For this review, take the finished solid that the model builds, in its own axes (mm). Face numbers are marked on the shaded views. A direction names the side the tool comes from. Give positions to 0.01 mm unless a question says otherwise; leave off trailing zeros. Write each loop counter-clockwise with the first axis right and the second up, starting at its lowest first coordinate (ties: lowest second). Pieces come first, ordered by that corner, then holes. Notation, with made-up numbers: (24.5, -28) -> (43.5, -28) arc R19 ccw to (43.5, -19) -> close; hole circle Ø5 at (39.25, 53.25). An arc over 180 degrees is marked (long way). Answer as CSV lines item,"result".
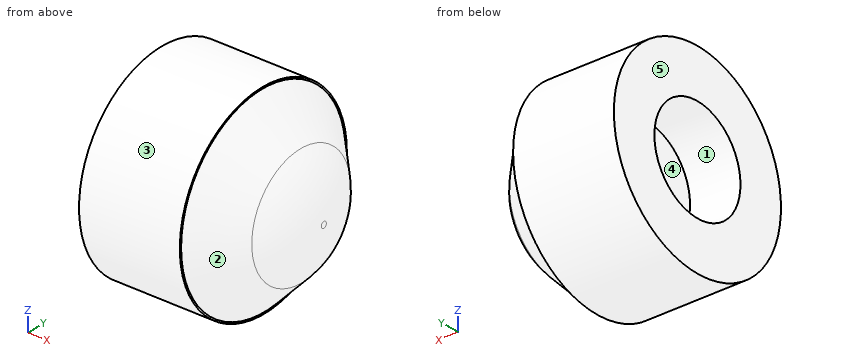
```python
from build123d import *

# Parameters (mm, degrees)
SKETCH020_R     = 9.9
PAD011_DEPTH    = 10
SKETCH021_R     = 9.75
PAD012_DEPTH    = 6
PAD012_TAPER    = 46
SKETCH022_R     = 5.09902
POCKET005_DEPTH = 25
FILLET_R        = 8


with BuildPart() as part:
    # Sketch020 → Pad011 (new body)
    with BuildSketch(Plane.YZ.offset(20)):
        Circle(SKETCH020_R)
    extrude(amount=PAD011_DEPTH)

    # Sketch021 → Pad012 (join)
    with BuildSketch(Plane.YZ.offset(30)):
        Circle(SKETCH021_R)
    extrude(amount=PAD012_DEPTH, taper=PAD012_TAPER)

    # Sketch022 → Pocket005 (cut)
    with BuildSketch(Plane.YZ):
        Circle(SKETCH022_R)
    extrude(amount=POCKET005_DEPTH, mode=Mode.SUBTRACT)

    # Fillet
    fillet_edges = [part.edges().sort_by_distance(p)[0] for p in [
        (36, -3.536818, 0),
    ]]
    fillet(fillet_edges, radius=FILLET_R)


with BuildPart() as part_1:
    # Body005 placement: moved
    add(part.part.moved(Location((0, 70, 20))))


solid = part_1.part
```
Q1. Add section B-B (x = 29.5). Write out the cut boundary in (y, z), plus the area to 3 significant figures.
Answer block:
outline,"circle Ø19.8 at (70, 20)"
area,"308 mm2"
Q2. Clearance check with flat-ended pins moving along their axes: pin 1 (8 mm diameter, centred on x = 26, y = 77, fed in from +Z); pin 2 (6 mm diameter, centred on y = 71, z = 16, fed in from +X); pin 3 (3 mm diameter, centred on x = 27.5, y = 64.5, fed in from -Z); pin 4 (6 mm diameter, centred on x = 25.5, y = 68, fed in from -Z). State where each tip first meets the part, or that it passes through.
Answer block:
pin 1,"stops at z = 29.43"
pin 2,"stops at x = 35.96"
pin 3,"stops at z = 10.94"
pin 4,"stops at z = 10.1"
Q3. To check wall thickness, follow probe 1 along Y at (x, z) = (22, 19.75); probe 2 along Z at (x, y) = (23.4, 70); probe 3 along X at (y, z) = (68, 19.25). State the ranges of each line that lie inside material, in increasing order. Write a range as [from, to].
Answer block:
probe 1,"y = [60.1, 64.91], [75.09, 79.9]"
probe 2,"z = [10.1, 14.9], [25.1, 29.9]"
probe 3,"x = [25, 35.79]"
Q4. Add section A-A (x = 24.25). Write out the cut boundary in (y, z), plus the area to 3 significant figures.
Answer block:
outline,"circle Ø19.8 at (70, 20); hole circle Ø10.2 at (70, 20)"
area,"226 mm2"
Q5. Draft analysis for pull direction Y (two halves, no side actions). For the marked faces 3, 4 and 5, state which applies: released by +Y, released by -Y, zero draft, split by the parting line, or undercut.
Answer block:
face 3,"split by the parting line"
face 4,"undercut"
face 5,"zero draft"
Q6. For the marked faces 1 and 2, list the 3-axis set-ups (+Z, -Z, +X, -X, +Y, -Y) from which the entire face can be reached by the end or side of a thin tool; tool diameter is ignored.
Answer block:
face 1,"-X"
face 2,"+X"
